Source: CAD feature listing. Evaluate the final solid. Frame: model axes, mm. A direction names the side the tool comes from. Give positions to 0.01 mm unless a question says otherwise; leave off trailing zeros. Order: outer loops, then holes, each group sorted by start corner. A loop starts at its lowest first (then second) coordinate and runs counter-clockwise, first axis right, second up. Notation, with made-up numbers: (54.25, 29.5) - (59.25, 29.5) arc R23 cw to (59.25, 56.5) - close; hole circle Ø10 at (82, -16). An arc over 180 degrees is marked (long way). Answer as CSV lines item,"result".
```python
from build123d import *

# Parameters (mm, degrees)
SKETCH1_R                         = 6.5
BOSS_EXTRUDE1_DEPTH               = 10
SKETCH2_R                         = 14
CUT_EXTRUDE1_DEPTH                = 14
CHAMFER1_SIZE                     = 1
CHAMFER2_SIZE                     = 4
FILLET1_R                         = 5
CUT_EXTRUDE2_DEPTH                = 4
FILLET2_R                         = 2
FILLET2_OF_MIRROR1_R              = 2
M10X1_25_TAPPED_HOLE1_D           = 8.8
M10X1_25_TAPPED_HOLE1_DEPTH       = 20
M10X1_25_TAPPED_HOLE1_CSINK_D     = 10
M10X1_25_TAPPED_HOLE1_CSINK_ANGLE = 90
M10X1_25_TAPPED_HOLE1_TIP         = 2.643786724


with BuildPart() as part:
    # Sketch1 → Boss-Extrude1 (new, symmetric)
    with BuildSketch(Plane.XY):
        with BuildLine():
            Line((-46, 0), (46, 0))
            Line((46, 0), (46, 15))
            Line((46, 15), (31.449256053, 74.112397284))
            ThreePointArc((31.449256053, 74.112397284), (30.363636327, 80.044097084), (30, 86.06334964))
            Line((30, 86.06334964), (30, 137))
            Line((30, 137), (16, 137))
            ThreePointArc((16, 137), (0, 145), (-16, 137))
            Line((-16, 137), (-30, 137))
            Line((-30, 137), (-30, 86.06334964))
            ThreePointArc((-30, 86.06334964), (-30.363636327, 80.044097084), (-31.449256053, 74.112397284))
            Line((-31.449256053, 74.112397284), (-46, 15))
            Line((-46, 15), (-46, 0))
        make_face()
        with Locations((0, 125)):
            Circle(SKETCH1_R, mode=Mode.SUBTRACT)
    extrude(amount=BOSS_EXTRUDE1_DEPTH, both=True)

    # Sketch2 → Cut-Extrude1 (cut)
    with BuildSketch(Plane.XY.offset(10)):
        with Locations((0, 125)):
            Circle(SKETCH2_R)
    extrude(amount=-CUT_EXTRUDE1_DEPTH, mode=Mode.SUBTRACT)

    # Chamfer1
    chamfer1_edges = [part.edges().sort_by_distance(p)[0] for p in [
        (-14, 125, 10),
    ]]
    chamfer(chamfer1_edges, length=CHAMFER1_SIZE)

    # Chamfer2
    chamfer2_edges = [part.edges().sort_by_distance(p)[0] for p in [
        (-30, 137, 0),
        (30, 137, 0),
    ]]
    chamfer(chamfer2_edges, length=CHAMFER2_SIZE)

    # Fillet1
    fillet1_edges = [part.edges().sort_by_distance(p)[0] for p in [
        (-16, 137, 0),
        (26, 137, 0),
    ]]
    fillet(fillet1_edges, radius=FILLET1_R)

    # Sketch3 → Cut-Extrude2 (cut)
    with BuildSketch(Plane.XY.offset(10)):
        with BuildLine():
            Line((-18, 92), (-18, 86.06334964))
            ThreePointArc((-18, 86.06334964), (-18.450909046, 78.59947647), (-19.797077506, 71.244168718))
            Line((-19.797077506, 71.244168718), (-29.971112298, 29.912152377))
            ThreePointArc((-29.971112298, 29.912152377), (-28.49970745, 23.065287193), (-22.202993266, 20))
            Line((-22.202993266, 20), (22.202993266, 20))
            ThreePointArc((22.202993266, 20), (28.49970745, 23.065287193), (29.971112298, 29.912152377))
            Line((29.971112298, 29.912152377), (19.797077506, 71.244168718))
            ThreePointArc((19.797077506, 71.244168718), (18.450909046, 78.59947647), (18, 86.06334964))
            Line((18, 86.06334964), (18, 92))
            ThreePointArc((18, 92), (15.656854249, 97.656854249), (10, 100))
            Line((10, 100), (-10, 100))
            ThreePointArc((-10, 100), (-15.656854249, 97.656854249), (-18, 92))
        make_face()
    cut_extrude2 = extrude(amount=-CUT_EXTRUDE2_DEPTH, mode=Mode.SUBTRACT)

    # Fillet2
    fillet2_edges = [part.edges().sort_by_distance(p)[0] for p in [
        (15.656854249, 97.656854249, 6),
        (18, 89.03167482, 6),
        (18.450909046, 78.59947647, 6),
        (24.884094902, 50.578160548, 6),
        (28.49970745, 23.065287193, 6),
        (0, 20, 6),
        (-28.49970745, 23.065287193, 6),
        (-24.884094902, 50.578160548, 6),
        (-18.450909046, 78.59947647, 6),
        (-18, 89.03167482, 6),
        (-15.656854249, 97.656854249, 6),
        (0, 100, 6),
    ]]
    fillet(fillet2_edges, radius=FILLET2_R)

    # Mirror1: Cut-Extrude2 across plane
    add(cut_extrude2.mirror(Plane.XY), mode=Mode.SUBTRACT)

    # Fillet2 of Mirror1
    fillet2_of_mirror1_edges = [part.edges().sort_by_distance(p)[0] for p in [
        (15.656854249, 97.656854249, -6),
        (18, 89.03167482, -6),
        (18.450909046, 78.59947647, -6),
        (24.884094902, 50.578160548, -6),
        (28.49970745, 23.065287193, -6),
        (0, 20, -6),
        (-28.49970745, 23.065287193, -6),
        (-24.884094902, 50.578160548, -6),
        (-18.450909046, 78.59947647, -6),
        (-18, 89.03167482, -6),
        (-15.656854249, 97.656854249, -6),
        (0, 100, -6),
    ]]
    fillet(fillet2_of_mirror1_edges, radius=FILLET2_OF_MIRROR1_R)

    # M10x1.25 Tapped Hole1
    with Locations(Plane(origin=(0, 0, 0), x_dir=(-1, 0, 0), z_dir=(0, -1, 0))):
        with Locations((-30, 0), (30, 0)):
            CounterSinkHole(M10X1_25_TAPPED_HOLE1_D / 2, M10X1_25_TAPPED_HOLE1_CSINK_D / 2, depth=M10X1_25_TAPPED_HOLE1_DEPTH, counter_sink_angle=M10X1_25_TAPPED_HOLE1_CSINK_ANGLE)
            with Locations((0, 0, -(M10X1_25_TAPPED_HOLE1_DEPTH + M10X1_25_TAPPED_HOLE1_TIP / 2))):  # 118° drill point
                Cone(0, M10X1_25_TAPPED_HOLE1_D / 2, M10X1_25_TAPPED_HOLE1_TIP, mode=Mode.SUBTRACT)


solid = part.part
```
(1) Access query for faces 1 (the cylindrical face through (-25.936, 10.436, 1.685)), 2 (the flat face through (30, 109, 0)), 3 (the cylindrical face through (24.26, 50.73, -6.6)), 4 (the flat face through (-24.813, 50.867, 9.014)). Directions: +Z, -Z, +X, -X, +Y, -Y. A direction counts if a zero-diameter tool reaches every point of the face in a straight line with its end or side. Return the directions, or none.
Completed:
face 1,"-Y"
face 2,"+Z, -Z, +X, +Y"
face 3,"-Z"
face 4,"+Z"
(2) Mould query, pull axis Y, two halves, no side actions, for faces 5 (the conical face through (-30.729, 22.185, -0.23)), 6 (the flat face through (-30, 110, 0)), 7 (the cylindrical face through (24.26, 50.73, 6.6)). Classes: released by +Y, released by -Y, zero draft, split by the parting line, or undercut.
Completed:
face 5,"released by -Y"
face 6,"zero draft"
face 7,"undercut"
(3) Cut plane B-B (x = 0). Return loops of the section in (y, z), then the cut area to 3 significant figures.
Completed:
outline,"(0, -10) - (20, -10) - (20, -8) arc R2 cw to (22, -6) - (98, -6) arc R2 cw to (100, -8) - (100, -10) - (118.5, -10) - (118.5, -4) - (111, -4) - (111, 9) - (110, 10) - (100, 10) - (100, 8) arc R2 cw to (98, 6) - (22, 6) arc R2 cw to (20, 8) - (20, 10) - (0, 10) - close; (131.5, -10) - (145, -10) - (145, 10) - (140, 10) - (139, 9) - (139, -4) - (131.5, -4) - close"
area,"1,790 mm²"
(4) Ray query, line 1 (Y direction, x = 0, z = -7.2); line 2 (Y direction, x = -3, z = -6.5); line 3 (Z direction, x = 30, y = 14.5). Return the intervals inside material, ascending. Write a range as from..to.
Completed:
line 1,"0..20.17, 99.83..118.5, 131.5..145"
line 2,"0..20.68, 99.32..119.23, 130.77..144.77"
line 3,"-10..-4.4, 4.4..10"
(5) Contact query for flat-ended pins moving along their axis: pin 1 (2 mm diameter, centred on y = 120.5, z = 6, fed in from +X); pin 2 (6.5 mm diameter, centred on x = 18.5, z = 5, fed in from +Y); pin 3 (10 mm diameter, centred on y = 28.5, z = 2.5, fed in from +X). Output: stop coordinate, or through.
Completed:
pin 1,"x = 30"
pin 2,"y = 137.94"
pin 3,"x = 43.91"
(6) Cut plane A-A (y = 125). Return loops of the section in (x, z).
Completed:
outline,"(-30, -10) - (-6.5, -10) - (-6.5, -4) - (-14, -4) - (-14, 9) - (-15, 10) - (-30, 10) - close; (6.5, -10) - (30, -10) - (30, 10) - (15, 10) - (14, 9) - (14, -4) - (6.5, -4) - close"
(7) Cut plane C-C (x = -37). Return loops of the section in (y, z).
Completed:
outline,"(0, -10) - (51.56, -10) - (51.56, 10) - (0, 10) - close"
